Part print with two shaded views. Sizes in mm from the minimum x, y, z corner. A direction names the side the tool comes from. Coordinates: 2 decimals unless noted, no trailing zeros. Write each loop counter-clockwise with the first axis right and the second up, starting at its lowest first coordinate (ties: lowest second). Pieces come first, ordered by that corner, then holes.
Q1. Band-saw the part on B-B, the plane y = 80. Write the cut outline in (x, z), plus the area to 3 significant figures.
Q2. Band-saw the part on D-D, the plane z = 67. Write the cut outline in (x, y).
Q3. Pull direction Y, two halves, no side cores. Call the marked faces 1, 2 and 3: released by +Y, released by -Y, zero draft, split by the parting line, or undercut.
Q4. Band-saw the part on C-C, the plane z = 48. Write the cut outline in (x, y), plus the area to 3 significant figures.
Q5. Which spindle directions (+Z, -Z, +X, -X, +Y, -Y) get a long thin tool onto all of the face, cutting with end or side? Do the marked faces 4, 5 and 6. Say none if no direction does.
Q6. Band-saw the part on A-A, the plane y = 43.5. Write the cut outline in (x, z), plus the area to 3 significant figures.
Q7. Drill centre lines: probe 1 along Y at (x, z) = (4.25, 43.5); probe 2 along X at (y, z) = (15, 74); probe 3 along Y at (x, z) = (18.5, 48). Where is each one in solid material? Low to high.
Q8. Pin check, flat tips, straight feed: P1, Ø10, axis at x = 4, z = 19.5, coming from the -Y side; P2, Ø5, axis at x = 12.5, z = 50, coming from the +Y side; P3, Ø9.5, axis at y = 6, z = 43.5, coming from the +X side. Stop position of each tip, or through.
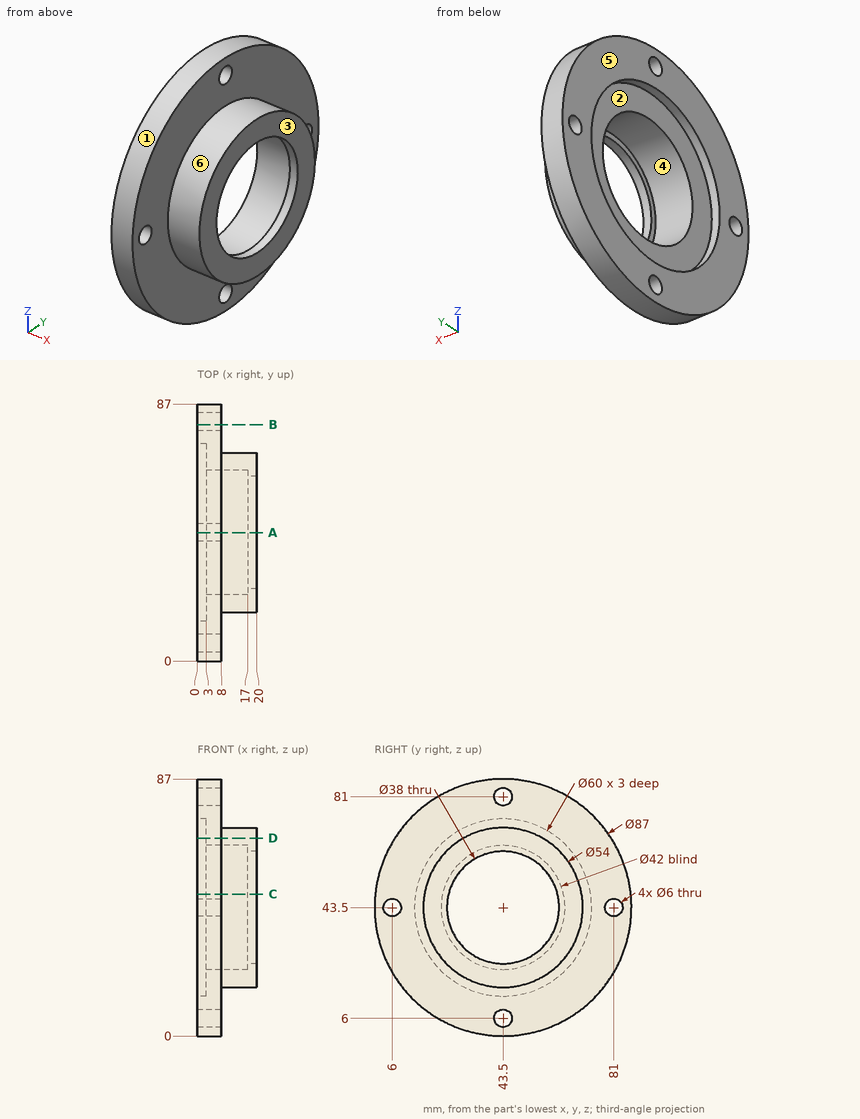
Answer sheet:
1. outline: (0, 19.84) - (8, 19.84) - (8, 40.67) - (0, 40.67) - close; (0, 46.33) - (8, 46.33) - (8, 67.16) - (0, 67.16) - close
1. area: 333 mm2
2. outline: (0, 6.89) - (8, 6.89) - (8, 30.21) - (20, 30.21) - (20, 56.79) - (8, 56.79) - (8, 80.11) - (0, 80.11) - (0, 62.15) - (3, 62.15) - (3, 24.85) - (0, 24.85) - close
3. face 1: split by the parting line
3. face 2: undercut
3. face 3: zero draft
4. outline: (0, 0.23) - (8, 0.23) - (8, 16.88) - (20, 16.88) - (20, 25.04) - (17, 25.04) - (17, 22.99) - (3, 22.99) - (3, 13.84) - (0, 13.84) - close; (0, 73.16) - (3, 73.16) - (3, 64.01) - (17, 64.01) - (17, 61.96) - (20, 61.96) - (20, 70.12) - (8, 70.12) - (8, 86.77) - (0, 86.77) - close
4. area: 468 mm2
5. face 4: -X
5. face 5: +Z, -Z, -X, +Y, -Y
5. face 6: +X
6. outline: (0, 0) - (8, 0) - (8, 3) - (0, 3) - close; (0, 9) - (8, 9) - (8, 16.5) - (20, 16.5) - (20, 24.5) - (17, 24.5) - (17, 22.5) - (3, 22.5) - (3, 13.5) - (0, 13.5) - close; (0, 73.5) - (3, 73.5) - (3, 64.5) - (17, 64.5) - (17, 62.5) - (20, 62.5) - (20, 70.5) - (8, 70.5) - (8, 78) - (0, 78) - close; (0, 84) - (8, 84) - (8, 87) - (0, 87) - close
6. area: 366 mm2
7. probe 1: y = 0 to 3, 9 to 22.5, 64.5 to 78, 84 to 87
7. probe 2: x = 0 to 8
7. probe 3: y = 16.88 to 25.04, 61.96 to 70.12
8. P1: stops at y = 4.37
8. P2: stops at y = 70.2
8. P3: stops at x = 8
